```python
from build123d import *

# Parameters (mm, degrees)
F0_R           = 5
F1_DEPTH       = 2.8
F2_D           = 3
F2_CSINK_D     = 7.5
F2_CSINK_ANGLE = 120
F5_R           = 5
F6_DEPTH       = 4
F7_D           = 3
F8_ANGLE       = 30
F10_ANGLE      = 180
F12_COUNT      = 4
F15_OFFSET     = 0.2
F16_D          = 1


with BuildPart() as f1:
    # F0 (on Top) → F1 (new body)
    with BuildSketch(Plane.XY):
        Circle(F0_R)
    extrude(amount=F1_DEPTH)

    # F2 (through all)
    with Locations(Plane(origin=(0, 0, 0), x_dir=(1, 0, 0), z_dir=(0, 0, -1))):
        with Locations((0, 0)):
            CounterSinkHole(F2_D / 2, F2_CSINK_D / 2, counter_sink_angle=F2_CSINK_ANGLE)


with BuildPart() as f6:
    # F5 (on Top) → F6 (new body)
    with BuildSketch(Plane.XY):
        with Locations((10.5, 0)):
            Circle(F5_R)
    extrude(amount=F6_DEPTH)

    # F7 (through all)
    with Locations(Plane(origin=(0, 0, 0), x_dir=(1, 0, 0), z_dir=(0, 0, -1))):
        with Locations((10.5, 0)):
            Hole(F7_D / 2)


with BuildPart() as f6_1:
    # F8: moved
    add(f6.part.rotate(Axis((0, 2.2134934552, 0), (0, 1, 0)), F8_ANGLE))


with BuildPart() as f6_2:
    # F9: moved
    add(f6_1.part.moved(Location((0.4, 0, 1.7))))


with BuildPart() as f1_1:
    # F10: moved
    add(f1.part.rotate(Axis((0, 2.2134934552, 0), (0, 1, 0)), F10_ANGLE))


with BuildPart() as f1_2:
    # F11: moved
    add(f1_1.part.moved(Location((0, 0, 2.8))))


with BuildPart() as f12_1:
    # F12: instance of F6
    add(f6_2.part.rotate(Axis((0, 0, 2.205231227), (0, 0, 1)), 1 * 360 / F12_COUNT))


with BuildPart() as f12_2:
    # F12: instance of F6
    add(f6_2.part.rotate(Axis((0, 0, 2.205231227), (0, 0, 1)), 2 * 360 / F12_COUNT))


with BuildPart() as f12_3:
    # F12: instance of F6
    add(f6_2.part.rotate(Axis((0, 0, 2.205231227), (0, 0, 1)), 3 * 360 / F12_COUNT))


with BuildPart() as f14:
    # F13 (on Front) → F14 (revolve)
    with BuildSketch(Plane.XZ):
        with BuildLine():
            Line((0, 4), (0, 0))
            Line((0, 0), (5.2, 0))
            Line((5.2, 0), (14.7262794416, -5.5))
            ThreePointArc((14.7262794416, -5.5), (15.4850984867, -5.5999004225), (16.0923048454, -5.1339745962))
            Line((16.0923048454, -5.1339745962), (16.5923048454, -4.2679491924))
            ThreePointArc((16.5923048454, -4.2679491924), (16.7921056904, -2.7503111022), (15.8602540378, -1.5358983849))
            Line((15.8602540378, -1.5358983849), (7.4320508076, 3.3301270189))
            ThreePointArc((7.4320508076, 3.3301270189), (6.2261460331, 3.8296291314), (4.9320508076, 4))
            Line((4.9320508076, 4), (0, 4))
        make_face()
    revolve(axis=Axis((0, 0, 2.205231227), (0, 0, 1)))

    # F15: cut F1, F6, F12_2, F12_1, F12_3, each made larger all round first
    f15_tool = offset(f1_2.part, amount=F15_OFFSET, kind=Kind.INTERSECTION, mode=Mode.PRIVATE)
    add(f15_tool, mode=Mode.SUBTRACT)
    f15_tool1 = offset(f6_2.part, amount=F15_OFFSET, kind=Kind.INTERSECTION, mode=Mode.PRIVATE)
    add(f15_tool1, mode=Mode.SUBTRACT)
    f15_tool2 = offset(f12_2.part, amount=F15_OFFSET, kind=Kind.INTERSECTION, mode=Mode.PRIVATE)
    add(f15_tool2, mode=Mode.SUBTRACT)
    f15_tool3 = offset(f12_1.part, amount=F15_OFFSET, kind=Kind.INTERSECTION, mode=Mode.PRIVATE)
    add(f15_tool3, mode=Mode.SUBTRACT)
    f15_tool4 = offset(f12_3.part, amount=F15_OFFSET, kind=Kind.INTERSECTION, mode=Mode.PRIVATE)
    add(f15_tool4, mode=Mode.SUBTRACT)

    # F16 (through all)
    with Locations(Plane(origin=(0, 0, 0), x_dir=(1, 0, 0), z_dir=(0, 0, -1))):
        with Locations((0, 0)):
            Hole(F16_D / 2)


solid = f14.part
```
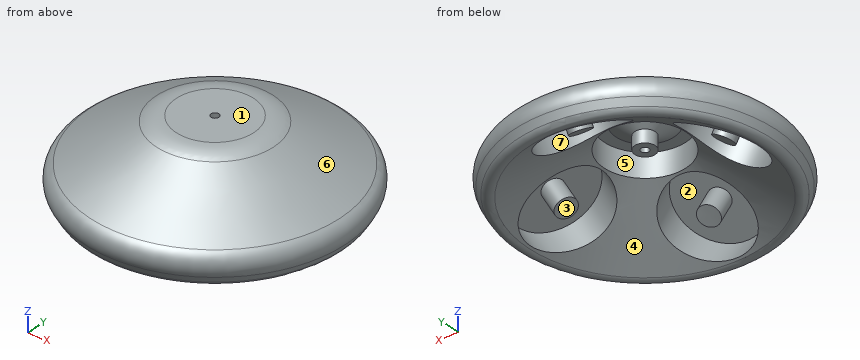
Input: part model. Units: mm. Frame: model coordinates. Face numbers are marked on the shaded views. A direction names the side the tool comes from. Round coordinates to 2 decimals unless told otherwise and drop trailing zeros. Write item = value, one per line.
(1) Access query for the marked faces 1, 2 and 3. Directions: +Z, -Z, +X, -X, +Y, -Y. A direction counts if a zero-diameter tool reaches every point of the face in a straight line with its end or side. Return the directions, or none.
Geometry check:
face_1 = +Z, +X, -X, +Y, -Y
face_2 = none
face_3 = -Z
(2) Contact query for flat-ended pins moving along their axis: pin 1 Ø3 at (y, z) = (-3.5, 2.5) entering from +X; pin 2 Ø4 at (x, y) = (4, -6.5) entering from -Z; pin 3 Ø4 at (y, z) = (-4.5, -4.5) entering from +X; pin 4 Ø4 at (x, z) = (-1, -3) entering from +Y. Output: stop coordinate, or through.
Geometry check:
pin_1 = 10.96
pin_2 = -2.56
pin_3 = 16.62
pin_4 = 16.86
(3) Section query A-A on z = -3. State how many separate pieces and enclosed holes the cut face has, then the cut area to 3 significant figures.
Geometry check:
separate_pieces = 5
enclosed_holes = 1
area = 368 mm^2
(4) Material intervals for probe 1 along Y at (x, z) = (0.5, -1.5); probe 2 along X at (y, z) = (9, -2); probe 3 along Y at (x, z) = (0, 2.75), sorted ascending.
Geometry check:
probe_1 = -15.79 to -14.34, -12.06 to -9.29, 9.29 to 12.06, 14.34 to 15.79
probe_2 = -13.72 to -5.06, -0.49 to 0.49, 5.06 to 13.72
probe_3 = -8.44 to -5.2, -3.26 to -0.5, 0.5 to 3.26, 5.2 to 8.44
(5) Pull-direction query (Z, two-part tool) for the marked faces 4, 5, 6 and 7; classes: +Z half, -Z half, draft (parallel to the pull), parting line (faces both ways), or undercut.
Geometry check:
face_4 = -Z half
face_5 = draft
face_6 = +Z half
face_7 = undercut
